Autodesk Fusion 360 part; units mm, degrees
sketch "Base" plane through (0, 0, 0) normal (0, 0, 1) x (1, 0, 0)
  line L0 (0, 0) -> (42, 0)
  line L1 (42, 0) -> (42, 42)
  line L2 (42, 42) -> (0, 42)
  line L3 (0, 42) -> (0, 0)
  dimension "d1" = 42
  dimension "d2" = 42
extrude "Extrude1" add sketch "Base" along normal blind 5
sketch "Mount holes" plane through (0, 0, 5) normal (0, 0, 1) x (-1, 0, 0)
  line L0 (0, -42) -> (0, 0)
  line L1 (0, 0) -> (-42, 0)
  line L2 (-42, 0) -> (-42, -42)
  line L3 (-42, -42) -> (0, -42)
  circle A0 centre (-3, -39) radius 1
  circle A1 centre (-39, -39) radius 1
  circle A2 centre (-3, -3) radius 1
  circle A3 centre (-39, -3) radius 1
  dimension "d8" = 2
  dimension "d9" = 3
  dimension "d10" = 3
  dimension "d11" = 2
  dimension "d12" = 3
  dimension "d13" = 3
  dimension "d14" = 2
  dimension "d15" = 3
  dimension "d16" = 3
  dimension "d17" = 2
  dimension "d18" = 3
  dimension "d19" = 3
extrude "Extrude2" cut sketch "Mount holes" against normal blind 5 contours A0 | A1 | A2 | A3
sketch "Motor holes" plane through (0, 0, 5) normal (0, 0, 1) x (-1, 0, 0)
  circle A0 centre (-39, -39) radius 1
  circle A1 centre (-3, -3) radius 1
  circle A2 centre (-3, -39) radius 1
  circle A3 centre (-39, -3) radius 1
  line L0 (0, -42) -> (0, 0)
  line L1 (0, 0) -> (-42, 0)
  line L2 (-42, 0) -> (-42, -42)
  line L3 (-42, -42) -> (0, -42)
  circle A4 centre (-12.25, -29.75) radius 1.25
  circle A5 centre (-29.75, -29.75) radius 1.25
  circle A6 centre (-12.25, -12.25) radius 1.25
  circle A7 centre (-29.75, -12.25) radius 1.25
  dimension "d22" = 2.5
  dimension "d23" = 2.5
  dimension "d25" = 12.25
  dimension "d27" = 2.5
  dimension "d28" = 2.5
  dimension "d30" = 12.25
  dimension "d31" = 12.25
  dimension "d32" = 12.25
  dimension "d33" = 12.25
  dimension "d34" = 12.25
  dimension "d35" = 12.25
  dimension "d36" = 12.25
extrude "Extrude3" cut sketch "Motor holes" against normal blind 5 contours A4 | A5 | A6 | A7
sketch "Fillets" plane through (0, 0, 5) normal (0, 0, 1) x (-1, 0, 0)
  circle A0 centre (-29.75, -29.75) radius 1.25
  circle A1 centre (-12.25, -12.25) radius 1.25
  circle A2 centre (-12.25, -29.75) radius 1.25
  circle A3 centre (-29.75, -12.25) radius 1.25
  circle A4 centre (-39, -39) radius 1
  circle A5 centre (-3, -3) radius 1
  circle A6 centre (-3, -39) radius 1
  circle A7 centre (-39, -3) radius 1
  line L0 (0, -42) -> (0, 0)
  line L1 (0, 0) -> (-42, 0)
  line L2 (-42, 0) -> (-42, -42)
  line L3 (-42, -42) -> (0, -42)
  circle A8 centre (-12.25, -29.75) radius 2.25
  circle A9 centre (-29.75, -29.75) radius 2.25
  circle A10 centre (-12.25, -12.25) radius 2.25
  circle A11 centre (-29.75, -12.25) radius 2.25
  dimension "d39" = 4.5
  dimension "d40" = 4.5
  dimension "d41" = 4.5
  dimension "d42" = 4.5
extrude "Extrude4" cut sketch "Fillets" against normal blind 2.5 contours A8 | A9 | A10 | A11
The model under review builds one solid part; all positions refer to its coordinate system, in mm. A direction names the side the tool comes from. Round coordinates to 2 decimals unless told otherwise and drop trailing zeros. Loops run counter-clockwise (first coordinate to the right, second up) from the corner with the lowest first, then second, coordinate; pieces in that order, holes last. Notation, with made-up numbers: M 31.25,-24 L 41.25,-24 A18 ccw 41.25,-20 Z; hole C 30.5,65.25 d5. An arc over 180 degrees is marked long. Answer as CSV lines item,"result". Start each with the question number.
Item 1: Mouldability with a two-part tool opening along Y and no side actions: class faces 3 (the face through (21, 0, 2)), 4 (the face through (38.46, 38.16, 2.54)), 5 (the face through (42, 21, 2)), 6 (the face through (3, 38, 3)) as released by +Y, released by -Y, zero draft, split by the parting line, or undercut.
Item 2: Consider section A-A (z = 3.5). State how many separate pieces and enclosed holes the cut face has, then the cut area to 3 significant figures.
Item 3: Wall thickness on line 1 (Y direction, x = 12.25, z = 3.35); line 2 (Y direction, x = 29.75, z = 1.2): over which ranges is each line inside the solid? List them lowest first. Write a range as [from, to].
Item 4: Consider section C-C (y = 12.25). Write out the cut boundary in (x, z), then the cut area to 3 significant figures.
Item 5: For faces 1 (the face through (27.67, 30.61, 3.77)), 2 (the face through (13.171, 28.905, 1.268)), list the 3-axis set-ups (+Z, -Z, +X, -X, +Y, -Y) from which the entire face can be reached by the end or side of a thin tool; tool diameter is ignored.
Item 6: Consider section B-B (x = 3). Write out the cut boundary in (y, z).
Item 7: Insertion check: P1, Ø2, axis at x = 13, y = 30, coming from the +Z side; P2, Ø1.5, axis at x = 12.25, y = 12.25, coming from the -Z side. Each pin has a flat end and moves straight along its axis. Give the tip position at first contact, or say it passes through.
Answer:
1,face 3,"released by -Y"
1,face 4,"undercut"
1,face 5,"zero draft"
1,face 6,"undercut"
2,separate pieces,"1"
2,enclosed holes,"8"
2,area,"1,690 mm^2"
3,line 1,"y = [0, 10], [14.5, 27.5], [32, 42]"
3,line 2,"y = [0, 11], [13.5, 28.5], [31, 42]"
4,outline,"M 0,0 L 11,0 L 11,2.5 L 10,2.5 L 10,5 L 0,5 Z; M 13.5,0 L 28.5,0 L 28.5,2.5 L 27.5,2.5 L 27.5,5 L 14.5,5 L 14.5,2.5 L 13.5,2.5 Z; M 31,0 L 42,0 L 42,5 L 32,5 L 32,2.5 L 31,2.5 Z"
4,area,"175 mm^2"
5,face 1,"+Z"
5,face 2,"+Z, -Z"
6,outline,"M 0,0 L 2,0 L 2,5 L 0,5 Z; M 4,0 L 38,0 L 38,5 L 4,5 Z; M 40,0 L 42,0 L 42,5 L 40,5 Z"
7,P1,"stops at z = 2.5"
7,P2,"passes through"
